from build123d import *

# Parameters (mm, degrees)
SKETCH1_R           = 5
BOSS_EXTRUDE1_DEPTH = 30
SKETCH2_W           = 20
SKETCH2_H           = 20
CUT_EXTRUDE1_DEPTH  = 25


with BuildPart() as part:
    # Sketch1 → Boss-Extrude1 (new body)
    with BuildSketch(Plane.XY):
        with BuildLine():
            Line((-10, 10), (10, 10))
            ThreePointArc((10, 10), (20, 0), (10, -10))
            Line((10, -10), (-10, -10))
            Line((-10, -10), (-10, 10))
        make_face()
        with Locations((10, 0)):
            Circle(SKETCH1_R, mode=Mode.SUBTRACT)
    extrude(amount=-BOSS_EXTRUDE1_DEPTH)

    # Sketch2 → Cut-Extrude1 (cut)
    with BuildSketch(Plane(origin=(20, 0, 0), x_dir=(0, 0, -1), z_dir=(1, 0, 0))):
        with Locations((15, 0)):
            Rectangle(SKETCH2_W, SKETCH2_H)
    extrude(amount=-CUT_EXTRUDE1_DEPTH, mode=Mode.SUBTRACT)


solid = part.part
CAD build for the part. Positions are in the model's coordinates, mm. A direction names the side the tool comes from. Coordinates: 2 decimals unless noted, no trailing zeros. Write each loop counter-clockwise with the first axis right and the second up, starting at its lowest first coordinate (ties: lowest second). Pieces come first, ordered by that corner, then holes. Notation, with made-up numbers: M -17,79 L 30,79 A20 ccw 30,86 Z; hole C 44.25,-17 d2. An arc over 180 degrees is marked long. Return JSON: item names as keys, results as strings.
Item 1: Drop flat-ended pins along their axis: pin 1 Ø1.5 at (y, z) = (-0.5, -7.5) entering from +X; pin 2 Ø6 at (x, y) = (10, -0.5) entering from -Z; pin 3 Ø8 at (y, z) = (-4.5, -23) entering from +X. Give the stop position or say it passes through.
Findings below:
{"pin 1": "stops at x = -5", "pin 2": "passes through", "pin 3": "stops at x = 19.95"}
Item 2: Which spindle directions (+Z, -Z, +X, -X, +Y, -Y) get a long thin tool onto all of the face, cutting with end or side? Do faces 4 (the flat face through (2, 0, 0)), 5 (the flat face through (5, -2, -25)). Say none if no direction does.
Findings below:
{"face 4": "+Z, +X, -X, +Y, -Y", "face 5": "+X, +Y, -Y"}
Item 3: Slice it at C-C, the plane z = -4.5. Write the cut outline in (x, y).
Findings below:
{"outline": "M -10,-10 L 10,-10 A10 ccw 10,10 L -10,10 Z; hole C 10,0 d10"}
Item 4: Slice it at D-D, the plane x = 14.25. Write the cut outline in (y, z).
Findings below:
{"outline": "M -9.05,-30 L -2.63,-30 L -2.63,-25 L -9.05,-25 Z; M -9.05,-5 L -2.63,-5 L -2.63,0 L -9.05,0 Z; M 2.63,-30 L 9.05,-30 L 9.05,-25 L 2.63,-25 Z; M 2.63,-5 L 9.05,-5 L 9.05,0 L 2.63,0 Z"}
Item 5: Two-plate mould, pull along X, no slides. Class faces 1 (the cylindrical face through (14.77, 1.5, -27.46)), 2 (the flat face through (-7, -10, -11)), 3 (the cylindrical face through (20, 0, -2)): +X half, -X half, draft (parallel to the pull), parting line (faces both ways), or undercut.
Findings below:
{"face 1": "undercut", "face 2": "draft", "face 3": "+X half"}
Item 6: Probe line 1 (Y direction, x = 10, z = -2.85); line 2 (Z direction, x = 11, y = 7.5); line 3 (X direction, y = -3, z = -20.5). List the from-to ranges inside material, lowest first. Write a range as from..to.
Findings below:
{"line 1": "y = -10..-5, 5..10", "line 2": "z = -30..-25, -5..0", "line 3": "x = -10..-5"}
Item 7: Slice it at B-B, the plane x = -1.25. Write the cut outline in (y, z), and give its area (3 significant figures).
Findings below:
{"outline": "M -10,-30 L 10,-30 L 10,-25 L -10,-25 Z; M -10,-5 L 10,-5 L 10,0 L -10,0 Z", "area": "200 mm2"}
Item 8: Slice it at A-A, the plane y = 0. Write the cut outline in (x, z), and give its area (3 significant figures).
Findings below:
{"outline": "M -10,-30 L 5,-30 L 5,-25 L -5,-25 L -5,-5 L 5,-5 L 5,0 L -10,0 Z; M 15,-30 L 20,-30 L 20,-25 L 15,-25 Z; M 15,-5 L 20,-5 L 20,0 L 15,0 Z", "area": "300 mm2"}
